Geometry: final body of the model. Coordinates: model frame, mm. Give positions to 0.01 mm unless a question says otherwise; leave off trailing zeros. Write each loop counter-clockwise with the first axis right and the second up, starting at its lowest first coordinate (ties: lowest second). Pieces come first, ordered by that corner, then holes. Notation, with made-up numbers: (47, 48.25) -> (102, 48.25) arc R18 cw to (102, 64.25) -> close; hole circle Ø10 at (-29, -22). An arc over 180 degrees is marked (long way). Answer as a JSON object with one key per item and string values.
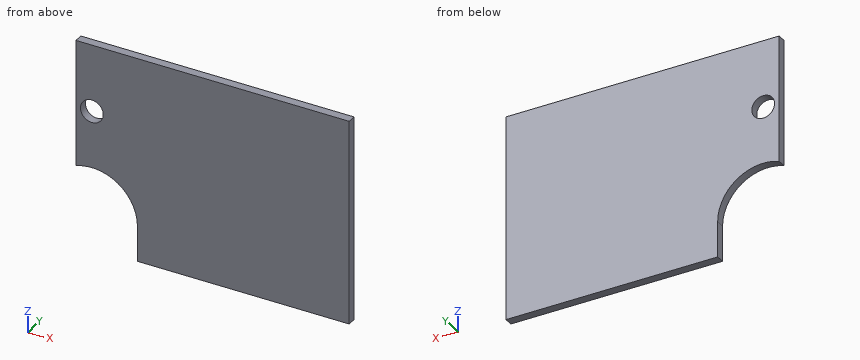
from build123d import *

# Parameters (mm, degrees)
SKETCH1_W           = 609.6
SKETCH1_H           = 457.2
BOSS_EXTRUDE1_DEPTH = 19.05
SKETCH2_R           = 25.4
CUT_EXTRUDE1_DEPTH  = 382.475952715
SKETCH4_R           = 101.6
CUT_EXTRUDE2_DEPTH  = 382.475952715
SKETCH6_W           = 137.16
SKETCH6_H           = 79.375
CUT_EXTRUDE3_DEPTH  = 382.475952715


with BuildPart() as part:
    # Sketch1 → Boss-Extrude1 (new body)
    with BuildSketch(Plane(origin=(0, 0, 0), x_dir=(1, 0, 0), z_dir=(0, 1, 0))):
        Rectangle(SKETCH1_W, SKETCH1_H)
    extrude(amount=BOSS_EXTRUDE1_DEPTH)

    # Sketch2 → Cut-Extrude1 (cut, through all)
    with BuildSketch(Plane.XZ):
        with Locations(Location((-269.24, 79.375, 0), (0, 0, 270))):
            Circle(SKETCH2_R)
    extrude(amount=-CUT_EXTRUDE1_DEPTH, mode=Mode.SUBTRACT)

    # Sketch4 → Cut-Extrude2 (cut, through all)
    with BuildSketch(Plane.XZ):
        with Locations((-269.24, -149.225)):
            Circle(SKETCH4_R)
    extrude(amount=-CUT_EXTRUDE2_DEPTH, mode=Mode.SUBTRACT)

    # Sketch6 → Cut-Extrude3 (cut, through all)
    with BuildSketch(Plane(origin=(0, 19.05, 0), x_dir=(1, 0, 0), z_dir=(0, 1, 0))):
        with Locations((-236.22, 188.9125)):
            Rectangle(SKETCH6_W, SKETCH6_H)
    extrude(amount=-CUT_EXTRUDE3_DEPTH, mode=Mode.SUBTRACT)


solid = part.part
Q1. Material intervals for L1, parallel to X at y = 7.75, z = -156.5; L2, parallel to X at y = 8, z = 74.5; L3, parallel to X at y = 18, z = 85, sorted ascending. Write a range as from..to.
Values:
{"L1": "-167.64..304.8", "L2": "-304.8..-294.17, -244.31..304.8", "L3": "-304.8..-294.01, -244.47..304.8"}
Q2. Cut plane A-A (x = -269.24). Return the cut outline in (y, z) (3 decimals), and give its area (3 significant figures).
Values:
{"outline": "(0, -47.625) -> (19.05, -47.625) -> (19.05, 53.975) -> (0, 53.975) -> close; (0, 104.775) -> (19.05, 104.775) -> (19.05, 228.6) -> (0, 228.6) -> close", "area": "4,290 mm²"}
Q3. Cut plane B-B (y = 4.25). Return the cut outline in (x, z) (3 decimals).
Values:
{"outline": "(-304.8, -54.051) arc R101.6 cw to (-167.64, -149.225) -> (-167.64, -228.6) -> (304.8, -228.6) -> (304.8, 228.6) -> (-304.8, 228.6) -> close; hole circle Ø50.8 at (-269.24, 79.375)"}
Q4. First-contact query: P1, Ø3, axis at y = 6, z = -88.5, coming from the -X side. Flat tip, straight axial feed; report the tip coordinate or a pass-through.
Values:
{"P1": "x = -188.92"}
Q5. Cut plane C-C (z = -84). Return the cut outline in (x, y), and give its area (3 significant figures).
Values:
{"outline": "(-191.34, 0) -> (304.8, 0) -> (304.8, 19.05) -> (-191.34, 19.05) -> close", "area": "9,450 mm²"}
